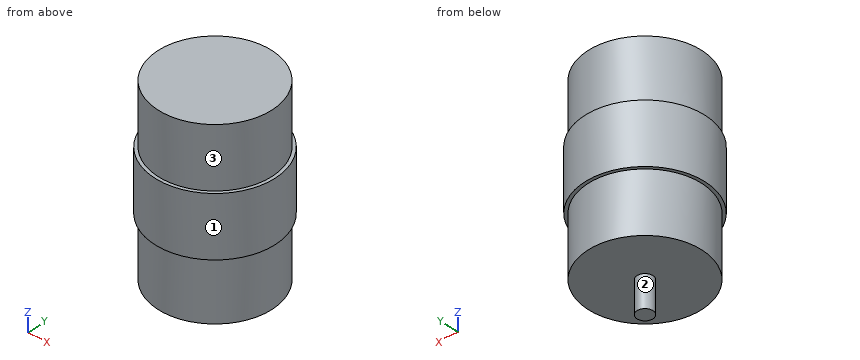
```python
from build123d import *

# Parameters (mm, degrees)
SKETCH1_R                = 19
SKETCH1_R_2              = 18
BOSS_EXTRUDE1_DEPTH      = 19
SKETCH1_3_R              = 18
BOSS_EXTRUDE2_DEPTH      = 38
BOSS_EXTRUDE2_DEPTH_BACK = 19
SKETCH2_R                = 2.5
BOSS_EXTRUDE3_DEPTH      = 10


with BuildPart() as part:
    # Sketch1 → Boss-Extrude1 (new body)
    with BuildSketch(Plane.XY):
        Circle(SKETCH1_R)
        Circle(SKETCH1_R_2, mode=Mode.SUBTRACT)
    extrude(amount=BOSS_EXTRUDE1_DEPTH)

    # Sketch1_3 → Boss-Extrude2 (add, two sides)
    with BuildSketch(Plane.XY) as boss_extrude2_sk:
        Circle(SKETCH1_3_R)
    extrude(amount=BOSS_EXTRUDE2_DEPTH)
    extrude(boss_extrude2_sk.sketch, amount=-BOSS_EXTRUDE2_DEPTH_BACK)

    # Sketch2 → Boss-Extrude3 (add)
    with BuildSketch(Plane(origin=(0, 0, -19), x_dir=(-1, 0, 0), z_dir=(0, 0, -1))):
        Circle(SKETCH2_R)
    extrude(amount=BOSS_EXTRUDE3_DEPTH)


solid = part.part
```
CAD build for the part. Positions are in the model's coordinates, mm. Face numbers are marked on the shaded views. A direction names the side the tool comes from. Round coordinates to 2 decimals unless told otherwise and drop trailing zeros. Write each loop counter-clockwise with the first axis right and the second up, starting at its lowest first coordinate (ties: lowest second). Pieces come first, ordered by that corner, then holes. Notation, with made-up numbers: (-10.5, 30) -> (37.5, 30) arc R7 cw to (37.5, 38) -> close; hole circle Ø2 at (33.25, 42.25). An arc over 180 degrees is marked (long way). Answer in a Markdown table with one row per item. Add a question column.
Item 1: Saw through at D-D, the plane x = -10.5. Write the cut outline in (y, z).
Item 2: Which spindle directions (+Z, -Z, +X, -X, +Y, -Y) get a long thin tool onto all of the face, cutting with end or side? Do the marked faces 1, 2 and 3. Say none if no direction does.
Item 3: Drill centre lines: line 1 (Z direction, x = -5, y = -1); line 2 (Y direction, x = 0, z = -1.5); line 3 (X direction, y = 0.5, z = 23). Where is each one in solid material? Low to high. Write a range as from..to.
Item 4: Drop flat-ended pins along their axis: pin 1 Ø5 at (y, z) = (4, -4.5) entering from -X; pin 2 Ø12 at (x, z) = (-11, 13) entering from -Y; pin 3 Ø6 at (x, y) = (2, 7) entering from -Z. Give the stop position or say it passes through.
Item 5: Saw through at C-C, the plane z = 24. Write the cut outline in (x, y).
Item 6: Saw through at A-A, the plane y = 0. Write the cut outline in (x, z).
Findings below:
| question | item | result |
|---|---|---|
| 1 | outline | (-15.84, 0) -> (-14.62, 0) -> (-14.62, -19) -> (14.62, -19) -> (14.62, 0) -> (15.84, 0) -> (15.84, 19) -> (14.62, 19) -> (14.62, 38) -> (-14.62, 38) -> (-14.62, 19) -> (-15.84, 19) -> close |
| 2 | face 1 | +Z, -Z |
| 2 | face 2 | -Z |
| 2 | face 3 | +Z |
| 3 | line 1 | z = -19..38 |
| 3 | line 2 | y = -18..18 |
| 3 | line 3 | x = -17.99..17.99 |
| 4 | pin 1 | stops at x = -17.94 |
| 4 | pin 2 | stops at y = -18.33 |
| 4 | pin 3 | stops at z = -19 |
| 5 | outline | circle Ø36 at (0, 0) |
| 6 | outline | (-19, 0) -> (-18, 0) -> (-18, -19) -> (-2.5, -19) -> (-2.5, -29) -> (2.5, -29) -> (2.5, -19) -> (18, -19) -> (18, 0) -> (19, 0) -> (19, 19) -> (18, 19) -> (18, 38) -> (-18, 38) -> (-18, 19) -> (-19, 19) -> close |
